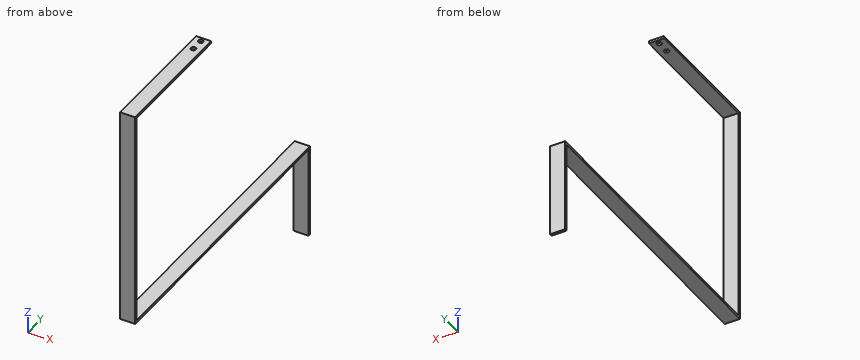
from build123d import *

# Parameters (mm, degrees)
CROQUIS1_W              = 38.1
CROQUIS1_H              = 6.31
SALIENTE_EXTRUIR1_DEPTH = 238.05
CROQUIS2_W              = 38.1
CROQUIS2_H              = 6.31
SALIENTE_EXTRUIR2_DEPTH = 755.1
CROQUIS3_W              = 38.1
CROQUIS3_H              = 6.31
SALIENTE_EXTRUIR3_DEPTH = 552.5
CROQUIS4_W              = 38.1
CROQUIS4_H              = 6.31
SALIENTE_EXTRUIR4_DEPTH = 314.39
CROQUIS6_W              = 38.1
CROQUIS6_H              = 6.31
SALIENTE_EXTRUIR5_DEPTH = 10
CROQUIS8_R              = 6.35
CORTAR_EXTRUIR1_DEPTH   = 10


with BuildPart() as part:
    # Croquis1 → Saliente-Extruir1 (new body)
    with BuildSketch(Plane.XY):
        Rectangle(CROQUIS1_W, CROQUIS1_H)
    extrude(amount=SALIENTE_EXTRUIR1_DEPTH)

    # Croquis2 → Saliente-Extruir2 (add)
    with BuildSketch(Plane.XZ.offset(3.155)):
        with Locations((0, 234.895)):
            Rectangle(CROQUIS2_W, CROQUIS2_H)
    extrude(amount=SALIENTE_EXTRUIR2_DEPTH)

    # Croquis3 → Saliente-Extruir3 (add)
    with BuildSketch(Plane.XY.offset(238.05)):
        with Locations((0, -755.1)):
            Rectangle(CROQUIS3_W, CROQUIS3_H)
    extrude(amount=SALIENTE_EXTRUIR3_DEPTH)

    # Croquis4 → Saliente-Extruir4 (add)
    with BuildSketch(Plane(origin=(0, -751.945, 0), x_dir=(1, 0, 0), z_dir=(0, 1, 0))):
        with Locations((0, -787.395)):
            Rectangle(CROQUIS4_W, CROQUIS4_H)
    extrude(amount=SALIENTE_EXTRUIR4_DEPTH)

    # Croquis6 → Saliente-Extruir5 (add)
    with BuildSketch(Plane(origin=(0, -437.555, 0), x_dir=(1, 0, 0), z_dir=(0, 1, 0))):
        with Locations((0, -787.395)):
            Rectangle(CROQUIS6_W, CROQUIS6_H)
    extrude(amount=SALIENTE_EXTRUIR5_DEPTH)

    # Croquis8 → Cortar-Extruir1 (cut)
    with BuildSketch(Plane.XY.offset(790.55)):
        with Locations((0, -471.447204666)):
            Circle(CROQUIS8_R)
        with Locations((0, -439.447204666)):
            Circle(CROQUIS8_R)
    extrude(amount=-CORTAR_EXTRUIR1_DEPTH, mode=Mode.SUBTRACT)


solid = part.part
Design review of the part built by this model. Coordinates are the model's own, in mm. Give positions to 0.01 mm unless a question says otherwise; leave off trailing zeros. Order: outer loops, then holes, each group sorted by start corner. A loop starts at its lowest first (then second) coordinate and runs counter-clockwise, first axis right, second up. Notation, with made-up numbers: (23, 26.25) - (36, 26.25) arc R16 ccw to (36, 31.25) - close; hole circle Ø1 at (-29.5, 9). An arc over 180 degrees is marked (long way). Use CSV: the item, a comma, the result in double quotes. Start each with the question number.
Q1. For line 1 (Y direction, x = 0, z = 789) (3 decimals); line 2 (Z direction, x = 12, y = -467.5); line 3 (Z direction, x = 4, y = -467.5), list the stretches that pass through material, from the lowest coordinate up.
Q2. Take a section at A-A (x = 0). State the section outline as (y, z) points (3 decimals).
Q3. For P1, Ø14.5, axis at x = 0, y = -471.45, coming from the -Z side; P2, Ø8, axis at x = -4.5, z = 148.5, coming from the -Y side (3 decimals); P3, Ø2, axis at x = 13, y = -177.5, coming from the +Z side, all flat-tipped, find the tip position at first contact; note any pin that passes through.
Q4. Take a section at B-B (z = 53.5). State the section outline as (x, y) points (3 decimals), and give its area (3 significant figures).
Calculated:
1,line 1,"y = -758.255 to -477.797, -465.097 to -445.797, -433.097 to -427.555"
1,line 2,"z = 231.74 to 238.05, 784.24 to 790.55"
1,line 3,"z = 231.74 to 238.05"
2,outline,"(-758.255, 231.74) - (-3.155, 231.74) - (-3.155, 0) - (3.155, 0) - (3.155, 238.05) - (-751.945, 238.05) - (-751.945, 784.24) - (-477.797, 784.24) - (-477.797, 790.55) - (-758.255, 790.55) - close; (-465.097, 784.24) - (-445.797, 784.24) - (-445.797, 790.55) - (-465.097, 790.55) - close; (-433.097, 784.24) - (-427.555, 784.24) - (-427.555, 790.55) - (-433.097, 790.55) - close"
3,P1,"stops at z = 231.74"
3,P2,"stops at y = -3.155"
3,P3,"stops at z = 238.05"
4,outline,"(-19.05, -3.155) - (19.05, -3.155) - (19.05, 3.155) - (-19.05, 3.155) - close"
4,area,"240 mm²"
